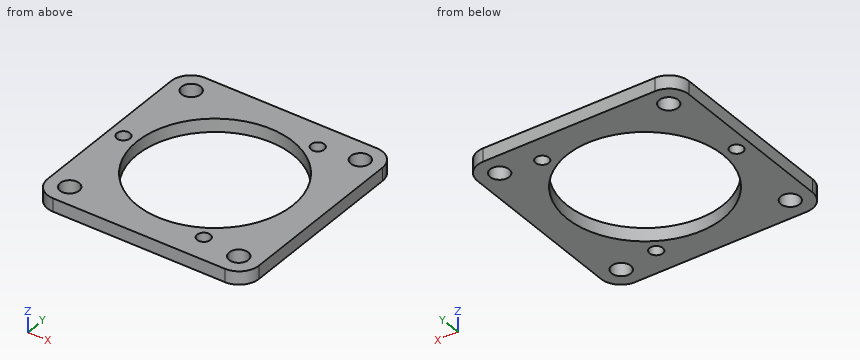
Autodesk Inventor part; units mm, degrees
ref_plane "YZ Plane" through (0, 0, 0) normal (1, 0, 0) x (0, 1, 0)
ref_plane "XZ Plane" through (0, 0, 0) normal (0, 1, 0) x (-1, 0, 0)
ref_plane "XY Plane" through (0, 0, 0) normal (0, 0, 1) x (1, 0, 0)
sketch "Sketch1" plane through (0, 0, 0) normal (0, 0, 1) x (1, 0, 0)
  line L0 (-13, 12) -> (13, 12)
  line L1 (13, 12) -> (13, -12)
  line L2 (13, -12) -> (-13, -12)
  line L3 (-13, -12) -> (-13, 12)
  line L4 (-13, 3.25) -> (-15, 3.25)
  line L5 (-15, 3.25) -> (-15, -3.25)
  line L6 (-15, -3.25) -> (-13, -3.25)
  line L7 (-13, -3.25) -> (-13, 3.25)
  line L8 (13, 3.25) -> (15, 3.25)
  line L9 (15, 3.25) -> (15, -3.25)
  line L10 (15, -3.25) -> (13, -3.25)
  line L11 (13, -3.25) -> (13, 3.25)
  line L12 (-25.4, 25.4) -> (25.4, 25.4)
  line L13 (25.4, 25.4) -> (25.4, -25.4)
  line L14 (25.4, -25.4) -> (-25.4, -25.4)
  line L15 (-25.4, -25.4) -> (-25.4, 25.4)
  circle A0 centre (0, 0) radius 7.1437
  circle A1 centre (-3, 12) radius 1.5
  line L16 (-13, 8) -> (-9, 12)
  line L17 (9, 12) -> (13, 8)
  line L18 (13, -8) -> (9, -12)
  line L19 (-13, -8) -> (-9, -12)
  circle A2 centre (0, 0) radius 18.7325
  circle A3 centre (-21.9964, 0) radius 1.5875
  circle A4 centre (11.0001, 19.0483) radius 1.5875
  circle A5 centre (11.0001, -19.0483) radius 1.5875
  circle A6 centre (0, 0) radius 21.9964 construction
  point P0 (-14, 3.25)
  point P1 (14, 3.25)
  point P2 (-14, -3.25)
  point P3 (14, -3.25)
  point P4 (-20.32, 20.32)
  point P5 (20.32, 20.32)
  point P6 (20.32, -20.32)
  point P7 (-20.32, -20.32)
  dimension "d0" = 24
  dimension "d1" = 12
  dimension "d2" = 26
  dimension "d3" = 13
  dimension "d4" = 2
  dimension "d5" = 6.5
  dimension "d6" = 3.25
  dimension "d7" = 2
  dimension "d8" = 14.2875
  dimension "d9" = 50.8
  dimension "d10" = 25.4
  dimension "d11" = 50.8
  dimension "d12" = 25.4
  dimension "d13" = 3
  dimension "d14" = 10
  dimension "d15" = 4
  dimension "d16" = 4
  dimension "d17" = 4
  dimension "d18" = 4
  dimension "d19" = 4
  dimension "d20" = 5.08
  dimension "d21" = 5.08
  dimension "d22" = 5.08
  dimension "d23" = 5.08
  dimension "d34" = 40.64
  dimension "d35" = 40.64
  dimension "d44" = 37.465
  dimension "d45" = 3.175
  dimension "d46" = 3.175
  dimension "d47" = 3.175
  dimension "d48" = 38.1
  dimension "d50" = 38.1
  dimension "d57" = 43.9928
  dimension "d58" = 38.0966
extrude "Extrusion1" add sketch "Sketch1" against normal blind 3.175 contours L0 L16 L3 | L0 L1 L17 | L19 L2 L3 | L18 L1 L2 | L12 L13 L14 L15 | A2 | A3 | A4 | A5
fillet "Fillet1" radius 3.175 4 edges at (-13, -3.25, -1.5875) (-13, 3.25, -1.5875) (13, 3.25, -1.5875) (13, -3.25, -1.5875)
hole "Hole1" at (-20.32, 20.32, 0) at (20.32, 20.32, 0) at (20.32, -20.32, 0) at (-20.32, -20.32, 0) direction (0, 0, -1) diameter 4.572 end through all
extrude "Extrusion2" cut sketch "Sketch1" against normal blind 25.4 contours L0 L16 L3 | L0 A1 L17 L1 L18 L2 L19 L3 L16 | L0 A1 | L0 L1 L17 | L19 L2 L3 | L18 L1 L2 | A0 | A2 | A3 | A4 | A5 picked at (-3.284, 11.1238)
fillet "Fillet2" radius 4.7625 4 edges at (25.4, 25.4, -1.5875) (-25.4, 25.4, -1.5875) (25.4, -25.4, -1.5875) (-25.4, -25.4, -1.5875)
equation "\"d7\" = d4"
equation "\"d16\" = d15"
equation "\"d17\" = d15"
equation "\"d18\" = d15"
equation "\"d19\" = d15"
equation "\"d46\" = d45"
equation "\"d47\" = d45"
properties part number "BD gearbox mount block"
Design review of the part built by this model. Coordinates are the model's own, in mm. Coordinates: 2 decimals unless noted, no trailing zeros. Loops run counter-clockwise (first coordinate to the right, second up) from the corner with the lowest first, then second, coordinate; pieces in that order, holes last. Notation, with made-up numbers: (24, -32.5) - (47, -32.5) arc R29 cw to (47, -5.5) - close; hole circle Ø8 at (-37.75, -27.5). An arc over 180 degrees is marked (long way). Use CSV: the item, a comma, the result in double quotes. Start each with the question number.
1. Clearance check with a flat-ended pin moving along its axis: pin 1 (3.5 mm diameter, centred on x = 11, y = -19.05, fed in from +Z). State where the tip first meets the part, or that it passes through.
2. Add section D-D on z = -2.15. Count the separate pieces of the cut face and the enclosed holes in it, plus the area to 3 significant figures.
3. Add section C-C on y = -16. Give the boundary of the cut face in (x, z) (3 decimals), plus the area to 3 significant figures.
4. Add section B-B on y = 0. Give the boundary of the cut face in (x, z) (1 decimal), plus the area to 3 significant figures.
5. To check wall thickness, follow probe 1 along X at (y, z) = (20.32, -1.5); probe 2 along Y at (x, z) = (12, -1.55); probe 3 along Y at (x, z) = (4, -0.7). State the ranges of each line that lie inside material, in increasing order.
6. Add section A-A on x = 0. Give the boundary of the cut face in (y, z) (1 decimal).
Resolved:
1,pin 1,"z = 0"
2,separate pieces,"1"
2,enclosed holes,"8"
2,area,"1,370 mm2"
3,outline,"(-25.4, -3.175) - (-9.742, -3.175) - (-9.742, 0) - (-25.4, 0) - close; (9.742, -3.175) - (25.4, -3.175) - (25.4, 0) - (9.742, 0) - close"
3,area,"99.4 mm2"
4,outline,"(-25.4, -3.2) - (-23.6, -3.2) - (-23.6, 0) - (-25.4, 0) - close; (-20.4, -3.2) - (-18.7, -3.2) - (-18.7, 0) - (-20.4, 0) - close; (18.7, -3.2) - (25.4, -3.2) - (25.4, 0) - (18.7, 0) - close"
4,area,"32.3 mm2"
5,probe 1,"-25.4 to -22.61, -18.03 to 10.05, 11.95 to 18.03, 22.61 to 25.4"
5,probe 2,"-25.4 to -20.28, -17.82 to -14.38, 14.38 to 17.82, 20.28 to 25.4"
5,probe 3,"-25.4 to -18.3, 18.3 to 25.4"
6,outline,"(-25.4, -3.2) - (-18.7, -3.2) - (-18.7, 0) - (-25.4, 0) - close; (18.7, -3.2) - (25.4, -3.2) - (25.4, 0) - (18.7, 0) - close"
